Input: part model. Units: mm. Frame: model coordinates. A direction names the side the tool comes from. Give positions to 0.01 mm unless a question says otherwise; leave off trailing zeros. Write each loop counter-clockwise with the first axis right and the second up, starting at its lowest first coordinate (ties: lowest second). Pieces come first, ordered by that corner, then holes. Notation, with made-up numbers: (16, 50) - (20, 50) arc R16 ccw to (20, 58) - close; hole circle Ø1 at (-13, 76). An arc over 180 degrees is marked (long way). Answer as CSV lines item,"result".
```python
from build123d import *

# Parameters (mm, degrees)
SKETCH021_W             = 14
SKETCH021_H             = 25
PAD015_DEPTH            = 3
SKETCH022_W             = 14
SKETCH022_H             = 7
PAD016_DEPTH            = 1.5
SKETCH023_W             = 1.8
SKETCH023_H             = 4
PAD017_DEPTH            = 1
SKETCH025_R             = 0.25
SKETCH027_R             = 0.25
BODY006_PLACEMENT_ANGLE = 180


with BuildPart() as part:
    # Sketch021 → Pad015 (new body)
    with BuildSketch(Plane.XY):
        Rectangle(SKETCH021_W, SKETCH021_H)
    extrude(amount=PAD015_DEPTH)

    # Sketch022 (on Face5 of Pad015) → Pad016 (join)
    with BuildSketch(Plane(origin=(0, 0, 0), x_dir=(1, 0, 0), z_dir=(0, 0, -1))):
        with Locations((0, 16)):
            Rectangle(SKETCH022_W, SKETCH022_H)
    extrude(amount=-PAD016_DEPTH)

    # Sketch023 (on Face11 of Pad016) → Pad017 (join)
    with BuildSketch(Plane.XY.offset(1.5)):
        with Locations((-3.5, -16)):
            Rectangle(SKETCH023_W, SKETCH023_H)
        with Locations((3.5, -16)):
            Rectangle(SKETCH023_W, SKETCH023_H)
    extrude(amount=PAD017_DEPTH)

    # AdditivePipe002: sweep along a path in Sketch024
    with BuildLine(Plane.XY.offset(1.5)) as additivepipe002_path:
        Line((3.652698, -18), (3.652698, -19.955732))
        ThreePointArc((3.652698, -19.955732), (3.7255554811, -20.1316255189), (3.901449, -20.204483))
        Line((3.901449, -20.204483), (5.252995, -20.204483))
        ThreePointArc((5.252995, -20.204483), (5.9787998058, -20.5051211942), (6.279438, -21.230926))
        Line((6.279438, -21.230926), (6.279438, -25.029842))
    # Sketch025 (on DatumPlane) → AdditivePipe002 (sweep)
    with BuildSketch(Plane(origin=(6.279438, -25.029842, 1.5), x_dir=(1, 0, 0), z_dir=(0, -1, 0))):
        Circle(SKETCH025_R)
    sweep(path=additivepipe002_path.line)

    # AdditivePipe003: sweep along a path in Sketch026
    with BuildLine(Plane.XY.offset(1.5)) as additivepipe003_path:
        Line((3.079145, -18), (1.9054359958, -20.158635665))
        ThreePointArc((1.9054359958, -20.158635665), (1.8760598704, -20.7128173949), (2.2882507497, -21.0844072569))
        Line((2.2882507497, -21.0844072569), (2.9810609114, -21.2900849643))
        ThreePointArc((2.9810609114, -21.2900849643), (3.3955781518, -21.5792681435), (3.554832, -22.0589447695))
        Line((3.554832, -22.0589447695), (3.554832, -25.04393))
    # Sketch027 (on DatumPlane) → AdditivePipe003 (sweep)
    with BuildSketch(Plane(origin=(3.554832, -25.04393, 1.5), x_dir=(1, 0, 0), z_dir=(0, -1, 0))):
        Circle(SKETCH027_R)
    sweep(path=additivepipe003_path.line)


with BuildPart() as part_1:
    # Body006 placement: moved
    add(part.part.moved(Location((-30.7, 3.7, 19.9))).rotate(Axis((-30.7, 3.7, 19.9), (0, 1, 0)), BODY006_PLACEMENT_ANGLE))


solid = part_1.part
```
Item 1: Cut plane C-C on z = 19. Return the cut outline in (x, y), plus the area to 3 significant figures.
The answers:
outline,"(-37.7, -15.8) - (-23.7, -15.8) - (-23.7, 16.2) - (-37.7, 16.2) - close"
area,"448 mm²"
Item 2: Cut plane B-B on y = -12.5. Return the cut outline in (x, z).
The answers:
outline,"(-37.7, 18.4) - (-35.1, 18.4) - (-35.1, 17.4) - (-33.3, 17.4) - (-33.3, 18.4) - (-28.1, 18.4) - (-28.1, 17.4) - (-26.3, 17.4) - (-26.3, 18.4) - (-23.7, 18.4) - (-23.7, 19.9) - (-37.7, 19.9) - close"
Item 3: Ray query, line 1 (Z direction, x = -34.25, y = -18.5); line 2 (Z direction, x = -33.5, y = -9); line 3 (Y direction, x = -34, z = 19.25). Return the intervals inside material, ascending. Write a range as from..to.
The answers:
line 1,"18.15..18.65"
line 2,"18.4..19.9"
line 3,"-15.8..16.2"
Item 4: Cut plane A-A on x = -29.75. Return the cut outline in (y, z).
The answers:
outline,"(-15.8, 18.4) - (-8.8, 18.4) - (-8.8, 16.9) - (16.2, 16.9) - (16.2, 19.9) - (-15.8, 19.9) - close"
Item 5: Contact query for flat-ended pins moving along their axis: pin 1 (0.7 mm diameter, centred on x = -33.5, y = -15, fed in from -Z); pin 2 (0.8 mm diameter, centred on x = -29.5, z = 19, fed in from -Y); pin 3 (1.4 mm diameter, centred on x = -34, y = -11.5, fed in from -Z). Output: stop coordinate, or through.
The answers:
pin 1,"z = 18.15"
pin 2,"y = -15.8"
pin 3,"z = 17.4"
Item 6: Reachability of faces 1 (the face through (-26.3, -12, 18)), 2 (the face through (-33.8, -15.2, 18.4)), 3 (the face through (-27, -12, 17.4)), 4 (the face through (-35.1, -12, 18)) from +Z, -Z, +X, -X, +Y, -Y: full face, straight path, thin tool, end or side. Return the list, or none.
The answers:
face 1,"-Z, +X, -Y"
face 2,"-Z"
face 3,"-Z, +X, -X, -Y"
face 4,"-Z, -X"
Item 7: Mould query, pull axis Y, two halves, no side actions, for faces 5 (the face through (-28.1, -12, 18)), 6 (the face through (-27, -10.3, 18)), 7 (the face through (-31, 16.2, 18)). Classes: +Y half, -Y half, draft (parallel to the pull), parting line (faces both ways), or undercut.
The answers:
face 5,"draft"
face 6,"undercut"
face 7,"+Y half"
